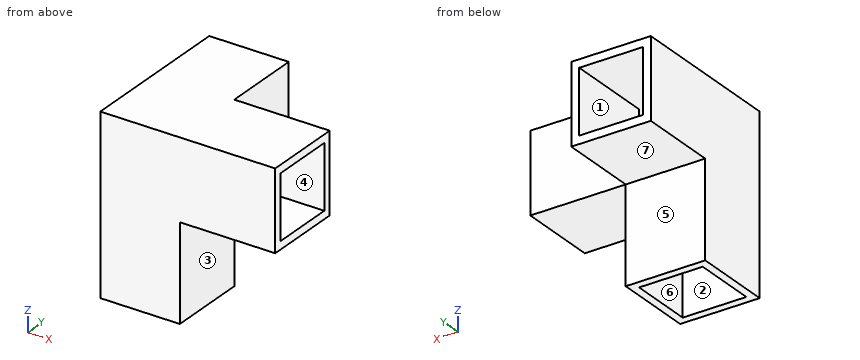
from build123d import *

# Parameters (mm, degrees)
BOSS_EXTRUDE1_DEPTH = 25
SKETCH3_W           = 25
SKETCH3_H           = 25
BOSS_EXTRUDE2_DEPTH = 25
SHELL2_T            = -2.5


with BuildPart() as part:
    # Sketch2 → Boss-Extrude1 (new body)
    with BuildSketch(Plane(origin=(0, 0, 0), x_dir=(1, 0, 0), z_dir=(0, 1, 0))):
        Polygon((0, 0), (30, 0), (30, -25), (-25, -25), (-25, 30), (0, 30), align=None)
    extrude(amount=BOSS_EXTRUDE1_DEPTH)

    # Sketch3 → Boss-Extrude2 (add)
    with BuildSketch(Plane(origin=(0, 25, 0), x_dir=(1, 0, 0), z_dir=(0, 1, 0))):
        with Locations((-12.5, -12.5)):
            Rectangle(SKETCH3_W, SKETCH3_H)
    extrude(amount=BOSS_EXTRUDE2_DEPTH)

    # Shell2
    shell2_openings = [part.faces().sort_by_distance(p)[0] for p in [
        (30, 12.5, 12.5),
        (-12.5, 12.5, -30),
        (-12.5, 50, 12.5),
    ]]
    offset(amount=SHELL2_T, openings=shell2_openings, kind=Kind.INTERSECTION)


solid = part.part
Model file for the job. Use its own axes, mm. Face numbers are marked on the shaded views. A direction names the side the tool comes from. Coordinates: 2 decimals unless noted, no trailing zeros. Order: outer loops, then holes, each group sorted by start corner. A loop starts at its lowest first (then second) coordinate and runs counter-clockwise, first axis right, second up. Notation, with made-up numbers: (-5.75, 32.25) -> (28.25, 32.25) arc R19 cw to (28.25, 44.25) -> close; hole circle Ø1 at (55.5, -33.5). An arc over 180 degrees is marked (long way). Return JSON: item names as keys, results as strings. Group by question number.
Item 1: Saw through at A-A on x = 24. Write the cut outline in (y, z).
Item 2: Flat gauge pins, fed straight in: P1, Ø20, axis at y = 13.5, z = -22.5, coming from the +X side; P2, Ø12.5, axis at x = -12.5, y = 35, coming from the -Z side; P3, Ø16, axis at x = -5, z = -10.5, coming from the +Y side. Where does each tip first touch, or does it go through?
Item 3: Tool access for the marked faces 1, 2, 3 and 4: list every direction of +Z, -Z, +X, -X, +Y, -Y with a clear straight run to the whole face (end or side of a thin tool).
Item 4: Saw through at C-C on z = 9.5. Write the cut outline in (x, y), then the cut area to 3 significant figures.
Item 5: Saw through at D-D on x = -6. Write the cut outline in (y, z).
Item 6: Wall check: line 1 along Z through (x, y) = (1, 17.5); line 2 along Z through (x, y) = (-1, 19.5). Give the ranges that are in metal, low to high. Write a range as [from, to].
Item 7: Saw through at B-B on y = 32.5. Write the cut outline in (x, z), then the cut area to 3 significant figures.
Item 8: Pull direction Y, two halves, no side cores. Call the marked faces 5, 6 and 7: pulls with the +Y half, pulls with the -Y half, needs draft (parallel to the pull), parting line crosses it, or undercut.
Values found:
{
 "1": {"outline": "(0, 0) -> (25, 0) -> (25, 25) -> (0, 25) -> close; hole (2.5, 2.5) -> (22.5, 2.5) -> (22.5, 22.5) -> (2.5, 22.5) -> close"},
 "2": {"P1": "stops at x = 0", "P2": "stops at z = 0", "P3": "stops at y = 25"},
 "3": {"face 1": "+Y", "face 2": "none", "face 3": "-Z, +X, +Y, -Y", "face 4": "+X"},
 "4": {"outline": "(-25, 0) -> (30, 0) -> (30, 2.5) -> (-22.5, 2.5) -> (-22.5, 50) -> (-25, 50) -> close; (-2.5, 22.5) -> (30, 22.5) -> (30, 25) -> (0, 25) -> (0, 50) -> (-2.5, 50) -> close", "area": "400 mm2"},
 "5": {"outline": "(0, -30) -> (2.5, -30) -> (2.5, 22.5) -> (50, 22.5) -> (50, 25) -> (0, 25) -> close; (22.5, -30) -> (25, -30) -> (25, 0) -> (50, 0) -> (50, 2.5) -> (22.5, 2.5) -> close"},
 "6": {"line 1": "z = [0, 2.5], [22.5, 25]", "line 2": "z = [-30, 2.5], [22.5, 25]"},
 "7": {"outline": "(-25, 0) -> (0, 0) -> (0, 25) -> (-25, 25) -> close; hole (-22.5, 2.5) -> (-2.5, 2.5) -> (-2.5, 22.5) -> (-22.5, 22.5) -> close", "area": "225 mm2"},
 "8": {"face 5": "pulls with the +Y half", "face 6": "undercut", "face 7": "needs draft"}
}
